Can you work these out from the model? Positions are in its coordinate system, mm. Face numbers are marked on the shaded views. A direction names the side the tool comes from. Give positions to 0.01 mm unless a question says otherwise; leave off trailing zeros. Write each loop counter-clockwise with the first axis right and the second up, starting at its lowest first coordinate (ties: lowest second). Pieces come first, ordered by that corner, then holes.
```python
from build123d import *

# Parameters (mm, degrees)
CROQUIS1_R              = 4.25
CROQUIS1_R_2            = 4.3
SALIENTE_EXTRUIR1_DEPTH = 12.5


with BuildPart() as part:
    # Croquis1 → Saliente-Extruir1 (new body)
    with BuildSketch(Plane.XY):
        with BuildLine():
            Line((-7.377684836, -5), (7.377684836, -5))
            ThreePointArc((7.377684836, -5), (9.051224581, -5.267438742), (10.558069892, -6.04311649))
            ThreePointArc((10.558069892, -6.04311649), (22.5, 0), (10.558069892, 6.04311649))
            ThreePointArc((10.558069892, 6.04311649), (9.051224581, 5.267438742), (7.377684836, 5))
            Line((7.377684836, 5), (-7.377684836, 5))
            ThreePointArc((-7.377684836, 5), (-9.051224581, 5.267438742), (-10.558069892, 6.04311649))
            ThreePointArc((-10.558069892, 6.04311649), (-22.5, 0), (-10.558069892, -6.04311649))
            ThreePointArc((-10.558069892, -6.04311649), (-9.051224581, -5.267438742), (-7.377684836, -5))
        make_face()
        with Locations((-15, 0)):
            Circle(CROQUIS1_R, mode=Mode.SUBTRACT)
        with Locations((15, 0)):
            Circle(CROQUIS1_R_2, mode=Mode.SUBTRACT)
    extrude(amount=SALIENTE_EXTRUIR1_DEPTH)


solid = part.part
```
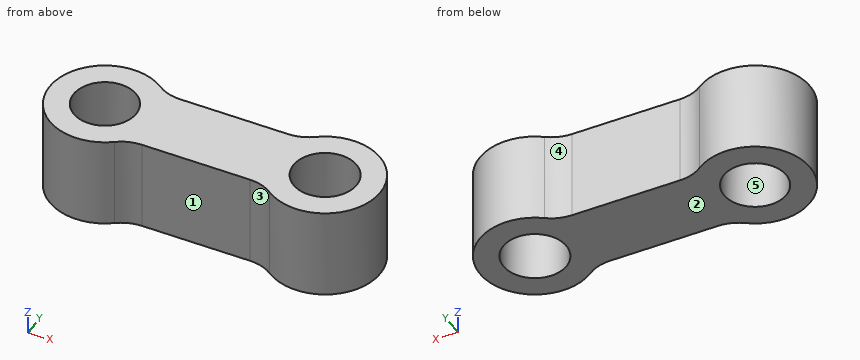
1) For pin 1 Ø6 at (x, y) = (5, 4.5) entering from -Z; pin 2 Ø7 at (x, y) = (15, 0) entering from -Z; pin 3 Ø6 at (x, z) = (2.5, 7) entering from +Y; pin 4 Ø1.5 at (y, z) = (-4, 1.5) entering from -X, each with a flat end and sliding along its axis, tell me the tip position at first contact or that it passes through.
Values follow:
pin 1: stops at z = 0
pin 2: passes through
pin 3: stops at y = 5
pin 4: stops at x = -21.76
2) For the marked faces 3, 4 and 5, which set-ups out of +Z, -Z, +X, -X, +Y, -Y let a thin tool reach every point of the face, with its end or its side?
Values follow:
face 3: +Z, -Z, -Y
face 4: +Z, -Z, +Y
face 5: +Z, -Z
3) Please list where these lines run through material, in increasing order: L1, parallel to X at y = -0.25, z = 10; L2, parallel to X at y = 3, z = 6.25; L3, parallel to Y at x = 15, z = 7.
Values follow:
L1: x = -22.5 to -19.24, -10.76 to 10.71, 19.29 to 22.5
L2: x = -21.87 to -18.01, -11.99 to 11.92, 18.08 to 21.87
L3: y = -7.5 to -4.3, 4.3 to 7.5
4) Suppose I cut it at B-B on x = 15. Write out the boundary of the cut face in (y, z).
Values follow:
outline: (-7.5, 0) - (-4.3, 0) - (-4.3, 12.5) - (-7.5, 12.5) - close; (4.3, 0) - (7.5, 0) - (7.5, 12.5) - (4.3, 12.5) - close
5) Suppose I cut it at C-C on z = 11.5. Write out the boundary of the cut face in (x, y), plus the area to 3 significant figures.
Values follow:
outline: (-10.56, -6.04) arc R5.37 cw to (-7.38, -5) - (7.38, -5) arc R5.37 cw to (10.56, -6.04) arc R7.5 ccw (long way) to (10.56, 6.04) arc R5.37 cw to (7.38, 5) - (-7.38, 5) arc R5.37 cw to (-10.56, 6.04) arc R7.5 ccw (long way) to start; hole circle Ø8.5 at (-15, 0); hole circle Ø8.6 at (15, 0)
area: 402 mm2
6) If we mould it in two halves opening along X, with no side actions, what happens to the marked faces 1 and 2? For each: +X half, -X half, draft (parallel to the pull), parting line (faces both ways), or undercut.
Values follow:
face 1: undercut
face 2: draft
7) Suppose I cut it at A-A on y = 0. Write out the boundary of the cut face in (x, z).
Values follow:
outline: (-22.5, 0) - (-19.25, 0) - (-19.25, 12.5) - (-22.5, 12.5) - close; (-10.75, 0) - (10.7, 0) - (10.7, 12.5) - (-10.75, 12.5) - close; (19.3, 0) - (22.5, 0) - (22.5, 12.5) - (19.3, 12.5) - close
8) Suppose I cut it at D-D on x = -3. Write out the boundary of the cut face in (y, z).
Values follow:
outline: (-5, 0) - (5, 0) - (5, 12.5) - (-5, 12.5) - close
